Study the drawing (mm; zero at the part's minimum x, y, z) and answer. Coordinates: 2 decimals unless noted, no trailing zeros. Loops run counter-clockwise (first coordinate to the right, second up) from the corner with the lowest first, then second, coordinate; pieces in that order, holes last. Notation, with made-up numbers: (7, -10.75) -> (12, -10.75) arc R28 cw to (12, 15.25) -> close; hole circle Ø2 at (-35, 22.5). An arc over 180 degrees is marked (long way). Answer in a Markdown table with one row per item.
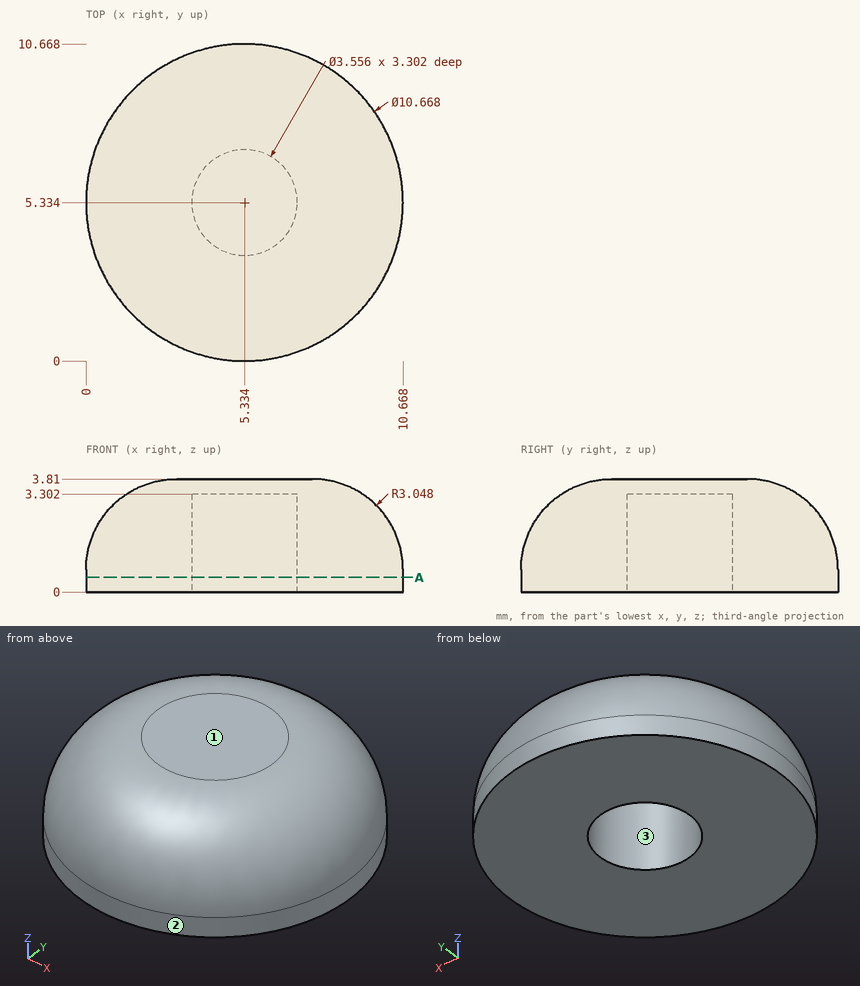
1. The mould has two halves that part along Y. Classify the marked faces 1, 2 and 3: pulls with the +Y half, pulls with the -Y half, needs draft (parallel to the pull), parting line crosses it, or undercut.
A:
| item | result |
|---|---|
| face 1 | needs draft |
| face 2 | parting line crosses it |
| face 3 | undercut |
2. Given pin 1 Ø2 at (x, z) = (9.5, 1.5) entering from -Y; pin 2 Ø1.8 at (x, y) = (5, 6) entering from -Z, each flat-ended and moving along its own axis, determine where each tip first touches the part or whether it passes through.
A:
| item | result |
|---|---|
| pin 1 | stops at y = 1.11 |
| pin 2 | stops at z = 3.3 |
3. Find the intervals of material crossed by probe 1 along Y at (x, z) = (5, 2.15); probe 2 along X at (y, z) = (4, 1.55); probe 3 along Y at (x, z) = (4.75, 1.7), in increasing order.
A:
| item | result |
|---|---|
| probe 1 | y = 0.35 to 3.59, 7.08 to 10.32 |
| probe 2 | x = 0.28 to 4.16, 6.51 to 10.39 |
| probe 3 | y = 0.18 to 3.65, 7.01 to 10.49 |
4. A cutting plane is placed at A-A on z = 0.5. Give the vertices of the cut face in (x, y).
A:
| item | result |
|---|---|
| outline | circle Ø10.67 at (5.33, 5.33); hole circle Ø3.56 at (5.33, 5.33) |
